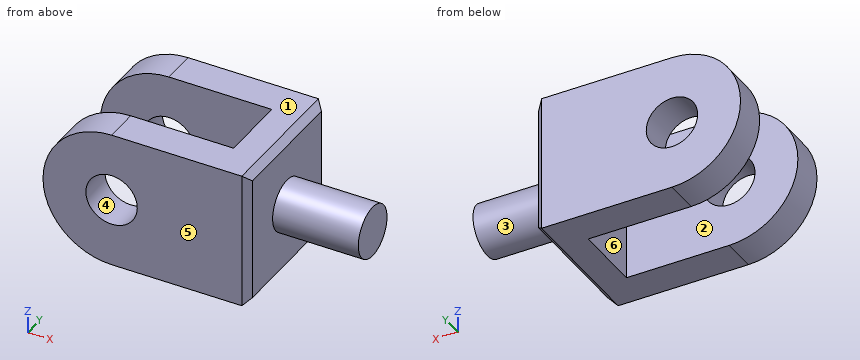
Autodesk Inventor part; units mm, degrees
ref_plane "YZ Plane" through (0, 0, 0) normal (1, 0, 0) x (0, 1, 0)
ref_plane "XZ Plane" through (0, 0, 0) normal (0, 1, 0) x (-1, 0, 0)
ref_plane "XY Plane" through (0, 0, 0) normal (0, 0, 1) x (1, 0, 0)
sketch "Skizze1" plane through (0, 0, 0) normal (0, 1, 0) x (-1, 0, 0)
  line L0 (0, 20) -> (40, 20)
  line L1 (40, -20) -> (0, -20)
  line L2 (0, -20) -> (0, 20)
  arc A0 (40, -20) -> (40, 20) centre (40, 0) ccw
  line L3 (0, 0) -> (81.992, 0) construction
  point P0 (20, -20)
  dimension "d0" = 40
  dimension "d2" = 40
  dimension "d3" = 20
extrude "Extrusion1" add sketch "Skizze1" along normal blind 40
sketch "Skizze2" plane through (0, 0, 0) normal (0, -1, 0) x (1, 0, 0)
  arc A0 (-40, 20) -> (-40, -20) centre (-40, 0) ccw
  point P0 (0, 0)
hole "Bohrung1" at (-40, 0, 0) direction (0, 1, 0) diameter 15 depth 40
sketch "Skizze3" plane through (-40, 0, 20) normal (0, 0, 1) x (1, 0, 0)
  line L0 (30, 10) -> (-20.9704, 10)
  line L1 (-20.9704, 10) -> (-20.9704, 30)
  line L2 (-20.9704, 30) -> (30, 30)
  line L3 (30, 30) -> (30, 10)
  line L4 (40, 0) -> (40, 40)
  point P0 (30, 20)
  point P1 (40, 20)
  dimension "d13" = 10
  dimension "d14" = 20
extrude "Extrusion2" cut sketch "Skizze3" against normal up to surface (40 mm away)
chamfer "Fasen1" distance 2 angle 45 4 edges at (0, 20, 20) (0, 40, 0) (0, 20, -20) (0, 0, 0)
sketch "Skizze4" plane through (0, 2, -18) normal (1, 0, 0) x (0, 0, -1)
  circle A0 centre (-18, 18) radius 7.5
  line L0 (0, 36) -> (0, 0)
  line L1 (-38, -2) -> (2, -2)
  point P0 (-18, -2)
  point P1 (0, 18)
  point P2 (-18, -2)
  dimension "d20" = 15
extrude "Extrusion3" add sketch "Skizze4" along normal blind 25
properties part number "6" material "Kupfer, Legierung"
Work out the finished part from the listing and answer in its coordinate system (mm). Face numbers are marked on the shaded views. A direction names the side the tool comes from. Coordinates: 2 decimals unless noted, no trailing zeros. Write each loop counter-clockwise with the first axis right and the second up, starting at its lowest first coordinate (ties: lowest second). Pieces come first, ordered by that corner, then holes.
Q1. Which of the six approach directions +Z, -Z, +X, -X, +Y, -Y give full straight-line access (tool end or side, diameter ignored) to the marked faces 1, 2 and 3?
Q2. A cutting plane is placed at D-D, the plane y = 15.5. Give the vertices of the cut face in (x, z).
Q3. A cutting plane is placed at A-A, the plane x = -14. Give the vertices of the cut face in (y, z), then the cut area to 3 significant figures.
Q4. Each of these flat-tipped pins is pushed along its axis until it touches: pin 1 Ø2 at (x, z) = (15.5, 6) entering from -Y; pin 2 Ø6 at (y, z) = (16.5, -13.5) entering from -X; pin 3 Ø2 at (y, z) = (35.5, 6.5) entering from -X; pin 4 Ø8 at (x, y) = (-43.5, 35.5) entering from -Z. Where does it stop, or does it pass through?
Q5. Determine the mould class of the marked faces 4, 5 and 6 for opening direction Y: released by +Y, released by -Y, zero draft, split by the parting line, or undercut.
Q6. A cutting plane is placed at C-C, the plane y = 5. Give the vertices of the cut face in (x, z), then the cut area to 3 significant figures.
Q7. Find the intervals of material crossed by line 1 (Z direction, x = -40, y = 3.5); line 2 (X direction, y = 8.25, z = 0); line 3 (Y direction, x = -55.5, z = 5.5), in increasing order.
Q8. A cutting plane is placed at B-B, the plane z = 0. Give the vertices of the cut face in (x, y), then the cut area to 3 significant figures.
Findings below:
1. face 1: +Z, +X, -X, +Y, -Y
1. face 2: +Z, -Z, -X
1. face 3: +X
2. outline: (-10, -20) - (-2, -20) - (0, -18) - (0, -6) - (25, -6) - (25, 6) - (0, 6) - (0, 18) - (-2, 20) - (-10, 20) - close
3. outline: (0, -20) - (10, -20) - (10, 20) - (0, 20) - close; (30, -20) - (40, -20) - (40, 20) - (30, 20) - close
3. area: 800 mm2
4. pin 1: stops at y = 14.41
4. pin 2: stops at x = -10
4. pin 3: stops at x = -59.23
4. pin 4: stops at z = -20
5. face 4: zero draft
5. face 5: released by -Y
5. face 6: undercut
6. outline: (-40, -20) - (-2, -20) - (0, -18) - (0, 18) - (-2, 20) - (-40, 20) arc R20 ccw to start; hole circle Ø15 at (-40, 0)
6. area: 2,050 mm2
7. line 1: z = -20 to -7.5, 7.5 to 20
7. line 2: x = -60 to -47.5, -32.5 to 0
7. line 3: y = 0 to 10, 30 to 40
8. outline: (-60, 0) - (-47.5, 0) - (-47.5, 10) - (-60, 10) - close; (-60, 30) - (-47.5, 30) - (-47.5, 40) - (-60, 40) - close; (-32.5, 0) - (-2, 0) - (0, 2) - (0, 12.5) - (25, 12.5) - (25, 27.5) - (0, 27.5) - (0, 38) - (-2, 40) - (-32.5, 40) - (-32.5, 30) - (-10, 30) - (-10, 10) - (-32.5, 10) - close
8. area: 1,470 mm2
